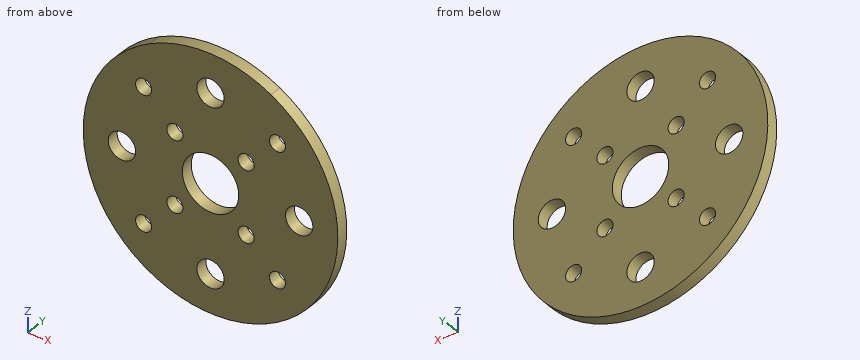
```python
from build123d import *
from build123d.topology import SkipClean

# Parameters (mm, degrees)
SKETCH1_R           = 0.85
SKETCH1_R_2         = 1.75
SKETCH1_R_3         = 0.5
SKETCH1_R_4         = 0.25
BOSS_EXTRUDE1_DEPTH = 0.75
BOSS_EXTRUDE4_START = -0.75
SKETCH5_R           = 0.25
SKETCH5_R_2         = 0.289113168
BOSS_EXTRUDE4_DEPTH = 0.75
CUT_EXTRUDE1_START  = -0.75
CUT_EXTRUDE1_DEPTH  = 0.75


with BuildPart() as part:
    # Sketch1 → Boss-Extrude1 (new body)
    with BuildSketch(Plane(origin=(0, 0, 0), x_dir=(1, 0, 0), z_dir=(0, 1, 0))):
        with BuildLine():
            Line((-3.75, -6.953236656), (-3.75, -14.65))
            Line((-3.75, -14.65), (3.75, -14.65))
            Line((3.75, -14.65), (3.75, -6.953236656))
            ThreePointArc((3.75, -6.953236656), (0, 7.9), (-3.75, -6.953236656))
        make_face()
        with Locations(Location((5.5, 0, 0), (0, 0, 270))):
            Circle(SKETCH1_R, mode=Mode.SUBTRACT)
        with Locations(Location((0, -5.5, 0), (0, 0, 270))):
            Circle(SKETCH1_R, mode=Mode.SUBTRACT)
        with Locations(Location((-5.5, 0, 0), (0, 0, 270))):
            Circle(SKETCH1_R, mode=Mode.SUBTRACT)
        with Locations(Location((0, 5.5, 0), (0, 0, 270))):
            Circle(SKETCH1_R, mode=Mode.SUBTRACT)
        with Locations(Location((0, 0, 0), (0, 0, 270))):
            Circle(SKETCH1_R_2, mode=Mode.SUBTRACT)
        with Locations(Location((-4.154, 4.154, 0), (0, 0, 270))):
            Circle(SKETCH1_R_3, mode=Mode.SUBTRACT)
        with Locations(Location((-2.21, 2.21, 0), (0, 0, 270))):
            Circle(SKETCH1_R_3, mode=Mode.SUBTRACT)
        with Locations(Location((4.154, 4.154, 0), (0, 0, 270))):
            Circle(SKETCH1_R_3, mode=Mode.SUBTRACT)
        with Locations(Location((2.21, 2.21, 0), (0, 0, 270))):
            Circle(SKETCH1_R_3, mode=Mode.SUBTRACT)
        with Locations(Location((4.154, -4.154, 0), (0, 0, 270))):
            Circle(SKETCH1_R_3, mode=Mode.SUBTRACT)
        with Locations(Location((2.21, -2.21, 0), (0, 0, 270))):
            Circle(SKETCH1_R_3, mode=Mode.SUBTRACT)
        with Locations(Location((-4.154, -4.154, 0), (0, 0, 270))):
            Circle(SKETCH1_R_3, mode=Mode.SUBTRACT)
        with Locations(Location((-2.21, -2.21, 0), (0, 0, 270))):
            Circle(SKETCH1_R_3, mode=Mode.SUBTRACT)
        with Locations(Location((-3, 0, 0), (0, 0, 270))):
            Circle(SKETCH1_R_4, mode=Mode.SUBTRACT)
        with Locations(Location((-1.5, -10.75, 0), (0, 0, 270))):
            Circle(SKETCH1_R_4, mode=Mode.SUBTRACT)
        with Locations(Location((3, 0, 0), (0, 0, 270))):
            Circle(SKETCH1_R_4, mode=Mode.SUBTRACT)
        with Locations(Location((1.5, -10.75, 0), (0, 0, 90))):
            Circle(SKETCH1_R_4, mode=Mode.SUBTRACT)
        with Locations(Location((-6.2, 2.25, 0), (0, 0, 270))):
            Circle(SKETCH1_R_4, mode=Mode.SUBTRACT)
        with Locations(Location((0, -9.75, 0), (0, 0, 270))):
            Circle(SKETCH1_R_4, mode=Mode.SUBTRACT)
        with Locations(Location((0, -7.75, 0), (0, 0, 270))):
            Circle(SKETCH1_R_4, mode=Mode.SUBTRACT)
        with Locations(Location((-1, -8.75, 0), (0, 0, 270))):
            Circle(SKETCH1_R_4, mode=Mode.SUBTRACT)
        with Locations(Location((1, -8.75, 0), (0, 0, 90))):
            Circle(SKETCH1_R_4, mode=Mode.SUBTRACT)
        with Locations(Location((-5.9, 3.55, 0), (0, 0, 270))):
            Circle(SKETCH1_R_4, mode=Mode.SUBTRACT)
        with Locations(Location((6.2, 2.25, 0), (0, 0, 270))):
            Circle(SKETCH1_R_4, mode=Mode.SUBTRACT)
        with Locations(Location((5.9, 3.55, 0), (0, 0, 270))):
            Circle(SKETCH1_R_4, mode=Mode.SUBTRACT)
    extrude(amount=BOSS_EXTRUDE1_DEPTH)

    # Sketch5 → Boss-Extrude4 (add)
    with BuildSketch(Plane(origin=(0, 0.75, 0), x_dir=(1, 0, 0), z_dir=(0, 1, 0)).offset(BOSS_EXTRUDE4_START)):
        with Locations((-5.9, 3.55)):
            Circle(SKETCH5_R)
        with Locations((-6.2, 2.25)):
            Circle(SKETCH5_R)
        with Locations((5.9, 3.55)):
            Circle(SKETCH5_R)
        with Locations((6.2, 2.25)):
            Circle(SKETCH5_R)
        with Locations((3, 0)):
            Circle(SKETCH5_R)
        with Locations((-3, 0)):
            Circle(SKETCH5_R_2)
        with Locations((0, -7.75)):
            Circle(SKETCH5_R)
    extrude(amount=BOSS_EXTRUDE4_DEPTH)

    # Sketch6 → Cut-Extrude1 (cut)
    with SkipClean():  # the faces are left unmerged after this step: merging them gives an invalid solid
        with BuildSketch(Plane(origin=(0, 0.75, 0), x_dir=(1, 0, 0), z_dir=(0, 1, 0)).offset(CUT_EXTRUDE1_START)):
            with BuildLine():
                ThreePointArc((3.75, -6.953236656), (0, -7.9), (-3.75, -6.953236656))
                Line((-3.75, -6.953236656), (-3.75, -14.65))
                Line((-3.75, -14.65), (3.75, -14.65))
                Line((3.75, -14.65), (3.75, -6.953236656))
            make_face()
        extrude(amount=CUT_EXTRUDE1_DEPTH, mode=Mode.SUBTRACT)


solid = part.part
```
Design review of the part built by this model. Coordinates are the model's own, in mm. Coordinates: 2 decimals unless noted, no trailing zeros. Write each loop counter-clockwise with the first axis right and the second up, starting at its lowest first coordinate (ties: lowest second). Pieces come first, ordered by that corner, then holes.
1) Add section D-D (y = 0.25). State how many separate pieces and enclosed holes the cut face has, plus the area to 3 significant figures.
2) Add section A-A (z = 0). Write out the cut boundary in (x, y).
3) Add section B-B (x = 0). Write out the cut boundary in (y, z), plus the area to 4 significant figures.
4) Add section C-C (x = 2.5). Write out the cut boundary in (y, z), plus the area to 3 significant figures.
5) To check wall thickness, follow L1, parallel to X at y = 0.65, z = 0; L2, parallel to Z at x = 0.75, y = 0.3; L3, parallel to X at y = 0.2, z = 2.21. State the ranges of each line that lie inside material, in increasing order.
Check result:
1. separate pieces: 1
1. enclosed holes: 13
1. area: 171 mm2
2. outline: (-7.9, 0) - (-6.35, 0) - (-6.35, 0.75) - (-7.9, 0.75) - close; (-4.65, 0) - (-1.75, 0) - (-1.75, 0.75) - (-4.65, 0.75) - close; (1.75, 0) - (4.65, 0) - (4.65, 0.75) - (1.75, 0.75) - close; (6.35, 0) - (7.9, 0) - (7.9, 0.75) - (6.35, 0.75) - close
3. outline: (0, -7.9) - (0.75, -7.9) - (0.75, -6.35) - (0, -6.35) - close; (0, -4.65) - (0.75, -4.65) - (0.75, -1.75) - (0, -1.75) - close; (0, 1.75) - (0.75, 1.75) - (0.75, 4.65) - (0, 4.65) - close; (0, 6.35) - (0.75, 6.35) - (0.75, 7.9) - (0, 7.9) - close
3. area: 6.675 mm2
4. outline: (0, -7.49) - (0.75, -7.49) - (0.75, -2.62) - (0, -2.62) - close; (0, -1.8) - (0.75, -1.8) - (0.75, 1.8) - (0, 1.8) - close; (0, 2.62) - (0.75, 2.62) - (0.75, 7.49) - (0, 7.49) - close
4. area: 10.0 mm2
5. L1: x = -7.9 to -6.35, -4.65 to -1.75, 1.75 to 4.65, 6.35 to 7.9
5. L2: z = -7.86 to -5.9, -5.1 to -1.58, 1.58 to 5.1, 5.9 to 7.86
5. L3: x = -7.58 to -2.71, -1.71 to 1.71, 2.71 to 7.58
